Check sheet for the modelled part. Datum: model origin and axes. Units: mm. Face numbers are marked on the shaded views. A direction names the side the tool comes from. Coordinates: 2 decimals unless noted, no trailing zeros. Loops run counter-clockwise (first coordinate to the right, second up) from the corner with the lowest first, then second, coordinate; pieces in that order, holes last. Notation, with made-up numbers: M 55.5,49.5 L 100.5,49.5 A16 ccw 100.5,68.5 Z; hole C -30.75,-39.5 d2. An arc over 180 degrees is marked long. Return JSON: item names as keys, results as strings.
from build123d import *

# Parameters (mm, degrees)
F0_W     = 20
F0_H     = 40
F0_R     = 5
F1_DEPTH = 15
F2_W     = 10
F2_H     = 25
F3_DEPTH = 20


with BuildPart() as f1:
    # F0 (on Front) → F1 (new body)
    with BuildSketch(Plane.XZ):
        with Locations((-0.241439, 0.093972)):
            Rectangle(F0_W, F0_H)
        with Locations((0, -8.363663)):
            Circle(F0_R, mode=Mode.SUBTRACT)
        with Locations((-0.175462, 8.823225)):
            Circle(F0_R, mode=Mode.SUBTRACT)
    extrude(amount=F1_DEPTH)

    # F2 (on Front) → F3 (join)
    with BuildSketch(Plane.XZ):
        with Locations((-15.241439, -7.406028)):
            Rectangle(F2_W, F2_H)
    extrude(amount=F3_DEPTH)


solid = f1.part
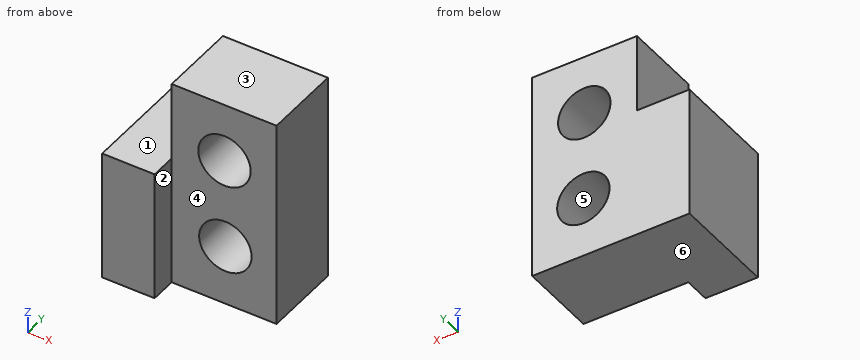
1) Go/stop test with flat-tipped pins: pin 1 Ø11.5 at (x, z) = (0, -8.36) entering from -Y; pin 2 Ø3 at (x, y) = (-14.5, -10) entering from +Z; pin 3 Ø1.5 at (y, z) = (-18, -8.5) entering from +X. Record where each tip stops, or that it passes through.
Answers:
{"pin 1": "y = -15", "pin 2": "z = 5.09", "pin 3": "x = -10.24"}
2) Section check D-D on z = -17. Record the cut outline in (x, y).
Answers:
{"outline": "M -20.24,-20 L -10.24,-20 L -10.24,-15 L 9.76,-15 L 9.76,0 L -20.24,0 Z"}
3) Scan lines: line 1 along Z through (x, y) = (0, -3); line 2 along Z through (x, y) = (-14.5, -2.5); line 3 along X through (y, z) = (-7.25, 14). Record each from-to range of solid material in increasing order. Write a range as [from, to].
Answers:
{"line 1": "[-19.91, -13.36], [-3.36, 3.83], [13.82, 20.09]", "line 2": "[-19.91, 5.09]", "line 3": "[-10.24, 9.76]"}
4) Section check A-A on x = 2.5. Record the cut outline in (y, z).
Answers:
{"outline": "M -15,-19.91 L 0,-19.91 L 0,-12.69 L -15,-12.69 Z; M -15,-4.03 L 0,-4.03 L 0,4.6 L -15,4.6 Z; M -15,13.05 L 0,13.05 L 0,20.09 L -15,20.09 Z"}
5) Section check B-B on z = 10. Record the cut outline in (x, y) (3 decimals).
Answers:
{"outline": "M -10.241,-15 L -5.035,-15 L -5.035,0 L -10.241,0 Z; M 4.684,-15 L 9.759,-15 L 9.759,0 L 4.684,0 Z"}
6) Section check C-C on y = -6.25. Record the cut outline in (x, z), then the cut area to 3 significant figures.
Answers:
{"outline": "M -20.24,-19.91 L 9.76,-19.91 L 9.76,20.09 L -10.24,20.09 L -10.24,5.09 L -20.24,5.09 Z; hole C -0.18,8.82 d10; hole C 0,-8.36 d10", "area": "893 mm²"}
7) Draft check along Z on the marked faces 4, 5 and 6. Enter one of: +Z half, -Z half, draft (parallel to the pull), parting line (faces both ways), or undercut.
Answers:
{"face 4": "draft", "face 5": "undercut", "face 6": "-Z half"}
8) Set-up check for the marked faces 1, 2 and 3: record each of +Z, -Z, +X, -X, +Y, -Y from which the full face is reachable in a straight line by a thin tool's end or side.
Answers:
{"face 1": "+Z, -X, +Y, -Y", "face 2": "+Z, -Z, +X, -Y", "face 3": "+Z, +X, -X, +Y, -Y"}
